```python
from build123d import *

# Parameters (mm, degrees)
F0_R     = 1.5
F0_R_2   = 2
F1_DEPTH = 5


with BuildPart() as f1:
    # F0 (on Top) → F1 (new body)
    with BuildSketch(Plane.XY):
        Polygon((57.630704, 133.314957), (-42.369296, 133.314957), (-42.369296, 103.314957), (-39.369296, 103.314957), (-39.369296, 88.314957), (-42.369296, 88.314957), (-42.369296, 48.314957), (-39.369296, 48.314957), (-39.369296, 33.314957), (-42.369296, 33.314957), (-42.369296, -21.685043), (-39.369296, -21.685043), (-39.369296, -36.685043), (-42.369296, -36.685043), (-42.369296, -66.685043), (57.630704, -66.685043), (57.630704, -36.685043), (54.630704, -36.685043), (54.630704, -21.685043), (57.630704, -21.685043), (57.630704, 33.314957), (54.630704, 33.314957), (54.630704, 48.314957), (57.630704, 48.314957), (57.630704, 88.314957), (54.630704, 88.314957), (54.630704, 103.314957), (57.630704, 103.314957), align=None)
        with Locations((-30.869296, -59.185043)):
            Circle(F0_R, mode=Mode.SUBTRACT)
        with Locations((-30.869296, 17.814957)):
            Circle(F0_R, mode=Mode.SUBTRACT)
        with Locations((46.130704, -59.185043)):
            Circle(F0_R, mode=Mode.SUBTRACT)
        with Locations((46.130704, 17.814957)):
            Circle(F0_R, mode=Mode.SUBTRACT)
        with Locations((7.630704, 83.314957)):
            Circle(F0_R_2, mode=Mode.SUBTRACT)
    extrude(amount=F1_DEPTH)


solid = f1.part
```
Could you check a few things on this model? Use its own coordinates, in mm. A direction names the side the tool comes from. Coordinates: 2 decimals unless noted, no trailing zeros. Loops run counter-clockwise (first coordinate to the right, second up) from the corner with the lowest first, then second, coordinate; pieces in that order, holes last.
1) Will these pins go through, and if not, where does the flat tip stop? pin 1 Ø1.5 at (y, z) = (99.5, 2.5) entering from +X; pin 2 Ø1.5 at (y, z) = (95.5, 2) entering from -X.
Reported:
pin 1: stops at x = 54.63
pin 2: stops at x = -39.37
2) Imagine slicing it at A-A (z = 2.7). State how many separate pieces and enclosed holes the cut face has, and give its area (3 significant figures).
Reported:
separate pieces: 1
enclosed holes: 5
area: 19,700 mm2
3) Which directions (+Z, -Z, +X, -X, +Y, -Y) give clear straight access to the entire face, cutting with the end or side of a thin tool? Please do faces 1 (the face through (-39.369, -29, 2)), 2 (the face through (54.631, 41, 2)), 3 (the face through (7, 35, 0)).
Reported:
face 1: +Z, -Z, -X
face 2: +Z, -Z, +X
face 3: -Z, +X, -X, +Y, -Y
4) Please list where these lines run through material, in increasing order: line 1 along X through (y, z) = (18, 0.2); line 2 along Y through (x, z) = (46, 1.95); line 3 along X through (y, z) = (36, 3.4).
Reported:
line 1: x = -42.37 to -32.36, -29.38 to 44.64, 47.62 to 57.63
line 2: y = -66.69 to -60.68, -57.69 to 16.32, 19.31 to 133.31
line 3: x = -39.37 to 54.63
5) Thinking about a two-plate mould opening in Y: for faces 4 (the face through (7, -66.685, 2)), 5 (the face through (-39.369, 41, 2)), 6 (the face through (8, 133.315, 2)), which applies, released by +Y, released by -Y, zero draft, split by the parting line, or undercut?
Reported:
face 4: released by -Y
face 5: undercut
face 6: released by +Y
6) Imagine slicing it at B-B (y = -33.5). List the corners of the cut face in (x, z) for me, and give its area (3 significant figures).
Reported:
outline: (-39.37, 0) - (54.63, 0) - (54.63, 5) - (-39.37, 5) - close
area: 470 mm2
